Can you work these out from the model? Positions are in its coordinate system, mm. Round coordinates to 2 decimals unless told otherwise and drop trailing zeros.
(1) Thinking about a two-plate mould opening in Z: for faces 1 (the face through (-182.545, 4.437, -238.07)), 2 (the face through (-62, 10, -4)), 3 (the face through (-289.05, 4.44, -8.67)), which applies, released by +Z, released by -Z, zero draft, split by the parting line, or undercut?
(2) I want a section at A-A on y = 6. Give the number of separate pieces and of enclosed holes in the cut face, plus the area to 3 significant figures.
(3) Will these pins go through, and if not, where does the flat tip stop? pin 1 Ø1.5 at (y, z) = (2, 167.5) entering from +X; pin 2 Ø6 at (x, z) = (-48, 52.5) entering from +Y; pin 3 Ø9.5 at (x, z) = (-72, -0.5) entering from +Y.
(4) If I drill on line 1 along X through (y, z) = (5.9, 0); line 2 along X through (y, z) = (2, 143.5); line 3 along Z through (x, y) = (-178, 7.25), over which ranges is the centre line in solid material (lowest first)?
from build123d import *

# Parameters (mm, degrees)
SKETCH2_R            = 300
SKETCH2_R_2          = 55
SKETCH2_R_3          = 40
BOSS_EXTRUDE10_DEPTH = 10
CHAMFER1_SIZE        = 1
SKETCH13_R           = 6
CUT_EXTRUDE1_DEPTH   = 7
SKETCH14_R           = 4
CUT_EXTRUDE2_DEPTH   = 3
CHAMFER2_SIZE        = 1


with BuildPart() as part:
    # Sketch2 → Boss-Extrude10 (new body)
    with BuildSketch(Plane(origin=(0, 0, 0), x_dir=(1, 0, 0), z_dir=(0, 1, 0))):
        with Locations(Location((0, 0, 0), (0, 0, 270))):
            Circle(SKETCH2_R)
        with Locations(Location((0, 0, 0), (0, 0, 270))):
            Circle(SKETCH2_R_2, mode=Mode.SUBTRACT)
        with Locations(Location((0, 250, 0), (0, 0, 270))):
            Circle(SKETCH2_R_3, mode=Mode.SUBTRACT)
        with Locations(Location((176.776695297, 176.776695297, 0), (0, 0, 270))):
            Circle(SKETCH2_R_3, mode=Mode.SUBTRACT)
        with Locations(Location((250, 0, 0), (0, 0, 270))):
            Circle(SKETCH2_R_3, mode=Mode.SUBTRACT)
        with Locations(Location((176.776695297, -176.776695297, 0), (0, 0, 270))):
            Circle(SKETCH2_R_3, mode=Mode.SUBTRACT)
        with Locations(Location((0, -250, 0), (0, 0, 270))):
            Circle(SKETCH2_R_3, mode=Mode.SUBTRACT)
        with Locations(Location((-176.776695297, -176.776695297, 0), (0, 0, 270))):
            Circle(SKETCH2_R_3, mode=Mode.SUBTRACT)
        with Locations(Location((-250, 0, 0), (0, 0, 270))):
            Circle(SKETCH2_R_3, mode=Mode.SUBTRACT)
        with Locations(Location((-176.776695297, 176.776695297, 0), (0, 0, 270))):
            Circle(SKETCH2_R_3, mode=Mode.SUBTRACT)
    extrude(amount=BOSS_EXTRUDE10_DEPTH)

    # Chamfer1
    chamfer1_edges = [part.edges().sort_by_distance(p)[0] for p in [
        (176.776695297, 10, -216.776695297),
        (250, 10, -40),
        (176.776695297, 10, 136.776695297),
        (0, 10, 210),
        (-176.776695297, 10, 136.776695297),
        (-250, 10, -40),
        (-176.776695297, 10, -216.776695297),
        (0, 10, -300),
        (0, 10, -290),
    ]]
    chamfer(chamfer1_edges, length=CHAMFER1_SIZE)

    # Sketch13 → Cut-Extrude1 (cut)
    with BuildSketch(Plane(origin=(0, 10, 0), x_dir=(1, 0, 0), z_dir=(0, 1, 0))):
        with Locations(Location((-71, 0, 0), (0, 0, 270))):
            Circle(SKETCH13_R)
        with Locations(Location((-50.204581464, 50.204581464, 0), (0, 0, 270))):
            Circle(SKETCH13_R)
        with Locations(Location((0, 71, 0), (0, 0, 270))):
            Circle(SKETCH13_R)
        with Locations(Location((50.204581464, 50.204581464, 0), (0, 0, 270))):
            Circle(SKETCH13_R)
        with Locations(Location((71, 0, 0), (0, 0, 270))):
            Circle(SKETCH13_R)
        with Locations(Location((50.204581464, -50.204581464, 0), (0, 0, 270))):
            Circle(SKETCH13_R)
        with Locations(Location((0, -71, 0), (0, 0, 270))):
            Circle(SKETCH13_R)
        with Locations(Location((-50.204581464, -50.204581464, 0), (0, 0, 270))):
            Circle(SKETCH13_R)
    extrude(amount=-CUT_EXTRUDE1_DEPTH, mode=Mode.SUBTRACT)

    # Sketch14 → Cut-Extrude2 (cut)
    with BuildSketch(Plane.XZ):
        with Locations(Location((-71, 0, 0), (0, 0, 270))):
            Circle(SKETCH14_R)
        with Locations(Location((-50.204581464, 50.204581464, 0), (0, 0, 270))):
            Circle(SKETCH14_R)
        with Locations(Location((0, 71, 0), (0, 0, 270))):
            Circle(SKETCH14_R)
        with Locations(Location((50.204581464, 50.204581464, 0), (0, 0, 270))):
            Circle(SKETCH14_R)
        with Locations(Location((71, 0, 0), (0, 0, 270))):
            Circle(SKETCH14_R)
        with Locations(Location((50.204581464, -50.204581464, 0), (0, 0, 270))):
            Circle(SKETCH14_R)
        with Locations(Location((0, -71, 0), (0, 0, 270))):
            Circle(SKETCH14_R)
        with Locations(Location((-50.204581464, -50.204581464, 0), (0, 0, 270))):
            Circle(SKETCH14_R)
    extrude(amount=-CUT_EXTRUDE2_DEPTH, mode=Mode.SUBTRACT)

    # Chamfer2
    chamfer2_edges = [part.edges().sort_by_distance(p)[0] for p in [
        (-71, 10, -6),
        (-50.204581464, 10, -56.204581464),
        (0, 10, -77),
        (50.204581464, 10, -56.204581464),
        (71, 10, -6),
        (50.204581464, 10, 44.204581464),
        (0, 10, 65),
        (-50.204581464, 10, 44.204581464),
    ]]
    chamfer(chamfer2_edges, length=CHAMFER2_SIZE)


solid = part.part
Filled sheet:
1. face 1: split by the parting line
1. face 2: zero draft
1. face 3: undercut
2. separate pieces: 1
2. enclosed holes: 17
2. area: 232,000 mm2
3. pin 1: stops at x = 249.39
3. pin 2: stops at y = 9.18
3. pin 3: stops at y = 3
4. line 1: x = -300 to -290, -210 to -77, -65 to -55, 55 to 65, 77 to 210, 290 to 300
4. line 2: x = -263.45 to -198.97, -154.58 to 154.58, 198.97 to 263.45
4. line 3: z = -241.49 to -216.76, -136.8 to 136.8, 216.76 to 241.49
